Geometry check sheet. Reference: the model listing, model coordinates, mm. A direction names the side the tool comes from. Coordinates: 2 decimals unless noted, no trailing zeros. Write each loop counter-clockwise with the first axis right and the second up, starting at its lowest first coordinate (ties: lowest second). Pieces come first, ordered by that corner, then holes. Notation, with made-up numbers: M 35.25,-25.5 L 88.25,-25.5 A19 cw 88.25,11.5 Z; hole C 67.5,-22.5 d1. An arc over 180 degrees is marked long. Write each question's results on one line, items separated by ' | '.
```python
from build123d import *

# Parameters (mm, degrees)
F0_W     = 85.6
F0_H     = 54
F0_R     = 1.45
F0_R_2   = 0.825
F0_R_3   = 0.445
F0_R_4   = 1.625
F0_R_5   = 1.15
F0_R_6   = 0.875
F0_R_7   = 0.46
F0_R_8   = 0.8
F1_DEPTH = 1.5
F3_DEPTH = 13
F4_R     = 4.15
F4_R_2   = 1.7
F5_DEPTH = 9.5
F6_R     = 0.5


with BuildPart() as f1:
    # F0 (on Top) → F1 (new body)
    with BuildSketch(Plane.XY):
        Rectangle(F0_W, F0_H)
        with Locations((-17.3, -9)):
            Circle(F0_R, mode=Mode.SUBTRACT)
        with Locations((30.375, -24.555)):
            Circle(F0_R_2, mode=Mode.SUBTRACT)
        with Locations((27.075, -21.255)):
            Circle(F0_R_3, mode=Mode.SUBTRACT)
        with Locations((33.425, -22.525)):
            Circle(F0_R_4, mode=Mode.SUBTRACT)
        with Locations((24.535, -19.985)):
            Circle(F0_R_3, mode=Mode.SUBTRACT)
        with Locations((24.535, -17.445)):
            Circle(F0_R_3, mode=Mode.SUBTRACT)
        with Locations((27.075, -18.715)):
            Circle(F0_R_3, mode=Mode.SUBTRACT)
        with Locations((24.535, -14.905)):
            Circle(F0_R_3, mode=Mode.SUBTRACT)
        with Locations((27.075, -16.175)):
            Circle(F0_R_3, mode=Mode.SUBTRACT)
        with Locations((27.075, -13.635)):
            Circle(F0_R_3, mode=Mode.SUBTRACT)
        with Locations((24.535, -12.365)):
            Circle(F0_R_3, mode=Mode.SUBTRACT)
        with Locations((30.375, -9.065)):
            Circle(F0_R_2, mode=Mode.SUBTRACT)
        with Locations((33.425, -11.095)):
            Circle(F0_R_4, mode=Mode.SUBTRACT)
        with Locations((32.65, -3.04)):
            Circle(F0_R_5, mode=Mode.SUBTRACT)
        with Locations((38.33, -3.04)):
            Circle(F0_R_5, mode=Mode.SUBTRACT)
        with Locations((-40.425, 23.375)):
            Circle(F0_R_6, mode=Mode.SUBTRACT)
        with Locations((-38.175, 23.375)):
            Circle(F0_R_6, mode=Mode.SUBTRACT)
        with Locations((-35.925, 23.375)):
            Circle(F0_R_6, mode=Mode.SUBTRACT)
        with Locations((-33.675, 23.375)):
            Circle(F0_R_6, mode=Mode.SUBTRACT)
        with Locations((-40.425, 25.625)):
            Circle(F0_R_6, mode=Mode.SUBTRACT)
        with Locations((-38.175, 25.625)):
            Circle(F0_R_6, mode=Mode.SUBTRACT)
        with Locations((-35.925, 25.625)):
            Circle(F0_R_6, mode=Mode.SUBTRACT)
        with Locations((-33.675, 25.625)):
            Circle(F0_R_6, mode=Mode.SUBTRACT)
        with Locations((-31.425, 23.375)):
            Circle(F0_R_6, mode=Mode.SUBTRACT)
        with Locations((-29.175, 23.375)):
            Circle(F0_R_6, mode=Mode.SUBTRACT)
        with Locations((-26.925, 23.375)):
            Circle(F0_R_6, mode=Mode.SUBTRACT)
        with Locations((-24.675, 23.375)):
            Circle(F0_R_6, mode=Mode.SUBTRACT)
        with Locations((-22.425, 23.375)):
            Circle(F0_R_6, mode=Mode.SUBTRACT)
        with Locations((-31.425, 25.625)):
            Circle(F0_R_6, mode=Mode.SUBTRACT)
        with Locations((-29.175, 25.625)):
            Circle(F0_R_6, mode=Mode.SUBTRACT)
        with Locations((-26.925, 25.625)):
            Circle(F0_R_6, mode=Mode.SUBTRACT)
        with Locations((-24.675, 25.625)):
            Circle(F0_R_6, mode=Mode.SUBTRACT)
        with Locations((-22.425, 25.625)):
            Circle(F0_R_6, mode=Mode.SUBTRACT)
        with Locations((-20.175, 23.375)):
            Circle(F0_R_6, mode=Mode.SUBTRACT)
        with Locations((-17.925, 23.375)):
            Circle(F0_R_6, mode=Mode.SUBTRACT)
        with Locations((-15.675, 23.375)):
            Circle(F0_R_6, mode=Mode.SUBTRACT)
        with Locations((-13.425, 23.375)):
            Circle(F0_R_6, mode=Mode.SUBTRACT)
        with Locations((-20.175, 25.625)):
            Circle(F0_R_6, mode=Mode.SUBTRACT)
        with Locations((-17.925, 25.625)):
            Circle(F0_R_6, mode=Mode.SUBTRACT)
        with Locations((-15.675, 25.625)):
            Circle(F0_R_6, mode=Mode.SUBTRACT)
        with Locations((-13.425, 25.625)):
            Circle(F0_R_6, mode=Mode.SUBTRACT)
        with Locations((33.01, 0.03)):
            Circle(F0_R_7, mode=Mode.SUBTRACT)
        with Locations((35.63, 0.03)):
            Circle(F0_R_7, mode=Mode.SUBTRACT)
        with Locations((33.01, 2.53)):
            Circle(F0_R_7, mode=Mode.SUBTRACT)
        with Locations((35.63, 2.53)):
            Circle(F0_R_7, mode=Mode.SUBTRACT)
        with Locations((33.01, 4.53)):
            Circle(F0_R_7, mode=Mode.SUBTRACT)
        with Locations((35.63, 4.53)):
            Circle(F0_R_7, mode=Mode.SUBTRACT)
        with Locations((33.01, 7.03)):
            Circle(F0_R_7, mode=Mode.SUBTRACT)
        with Locations((35.63, 7.03)):
            Circle(F0_R_7, mode=Mode.SUBTRACT)
        with Locations((32.65, 10.1)):
            Circle(F0_R_5, mode=Mode.SUBTRACT)
        with Locations((38.33, 10.1)):
            Circle(F0_R_5, mode=Mode.SUBTRACT)
        with BuildLine():
            Line((2.425, 18.3), (2.425, 16.3))
            ThreePointArc((2.425, 16.3), (1.05, 14.925), (-0.325, 16.3))
            Line((-0.325, 16.3), (-0.325, 18.3))
            ThreePointArc((-0.325, 18.3), (1.05, 19.675), (2.425, 18.3))
        make_face(mode=Mode.SUBTRACT)
        with BuildLine():
            ThreePointArc((7.175, 18.3), (8.55, 19.675), (9.925, 18.3))
            Line((9.925, 18.3), (9.925, 16.3))
            ThreePointArc((9.925, 16.3), (8.55, 14.925), (7.175, 16.3))
            Line((7.175, 16.3), (7.175, 18.3))
        make_face(mode=Mode.SUBTRACT)
        with Locations((18.2, 19)):
            Circle(F0_R_8, mode=Mode.SUBTRACT)
        with Locations((20.7, 19)):
            Circle(F0_R_8, mode=Mode.SUBTRACT)
        with BuildLine():
            Line((3.8, 22.5), (5.8, 22.5))
            ThreePointArc((5.8, 22.5), (7.3, 21), (5.8, 19.5))
            Line((5.8, 19.5), (3.8, 19.5))
            ThreePointArc((3.8, 19.5), (2.3, 21), (3.8, 22.5))
        make_face(mode=Mode.SUBTRACT)
        with Locations((18.2, 24)):
            Circle(F0_R_8, mode=Mode.SUBTRACT)
        with Locations((23.2, 19)):
            Circle(F0_R_8, mode=Mode.SUBTRACT)
        with Locations((25.7, 19)):
            Circle(F0_R_8, mode=Mode.SUBTRACT)
        with Locations((28.2, 19)):
            Circle(F0_R_8, mode=Mode.SUBTRACT)
        with Locations((37.8, 14.5)):
            Circle(F0_R, mode=Mode.SUBTRACT)
        with Locations((23.2, 24)):
            Circle(F0_R_8, mode=Mode.SUBTRACT)
        with Locations((28.2, 24)):
            Circle(F0_R_8, mode=Mode.SUBTRACT)
    extrude(amount=F1_DEPTH)

    # F2 (on face) → F3 (join)
    with BuildSketch(Plane.XY.offset(1.5)):
        with BuildLine():
            ThreePointArc((2.425, 16.3), (2.1694873279, 15.5016434865), (1.4979118217, 15))
            Line((1.4979118217, 15), (8.1020881783, 15))
            ThreePointArc((8.1020881783, 15), (7.4305126721, 15.5016434865), (7.175, 16.3))
            Line((7.175, 16.3), (7.175, 18.3))
            ThreePointArc((7.175, 18.3), (8.256849015, 19.6433865788), (9.8, 18.8728219619))
            Line((9.8, 18.8728219619), (9.8, 25))
            Line((9.8, 25), (-0.2, 25))
            Line((-0.2, 25), (-0.2, 18.8728219619))
            ThreePointArc((-0.2, 18.8728219619), (1.343150985, 19.6433865788), (2.425, 18.3))
            Line((2.425, 18.3), (2.425, 16.3))
        make_face()
        with BuildLine():
            ThreePointArc((3.8, 19.5), (2.3, 21), (3.8, 22.5))
            Line((3.8, 22.5), (5.8, 22.5))
            ThreePointArc((5.8, 22.5), (7.3, 21), (5.8, 19.5))
            Line((5.8, 19.5), (3.8, 19.5))
        make_face(mode=Mode.SUBTRACT)
        with BuildLine():
            Line((5.8, 22.5), (3.8, 22.5))
            ThreePointArc((3.8, 22.5), (2.3, 21), (3.8, 19.5))
            Line((3.8, 19.5), (5.8, 19.5))
            ThreePointArc((5.8, 19.5), (7.3, 21), (5.8, 22.5))
        make_face()
        with BuildLine():
            ThreePointArc((7.175, 16.3), (7.4305126721, 15.5016434865), (8.1020881783, 15))
            Line((8.1020881783, 15), (8.9979118217, 15))
            ThreePointArc((8.9979118217, 15), (9.4735383659, 15.2813234632), (9.8, 15.7271780381))
            Line((9.8, 15.7271780381), (9.8, 18.8728219619))
            ThreePointArc((9.8, 18.8728219619), (8.256849015, 19.6433865788), (7.175, 18.3))
            Line((7.175, 18.3), (7.175, 16.3))
        make_face()
        with BuildLine():
            ThreePointArc((-0.2, 15.7271780381), (0.1264616341, 15.2813234632), (0.6020881783, 15))
            Line((0.6020881783, 15), (1.4979118217, 15))
            ThreePointArc((1.4979118217, 15), (2.1694873279, 15.5016434865), (2.425, 16.3))
            Line((2.425, 16.3), (2.425, 18.3))
            ThreePointArc((2.425, 18.3), (1.343150985, 19.6433865788), (-0.2, 18.8728219619))
            Line((-0.2, 18.8728219619), (-0.2, 15.7271780381))
        make_face()
        with BuildLine():
            Line((-0.2, 15.7271780381), (-0.2, 15))
            Line((-0.2, 15), (0.6020881783, 15))
            ThreePointArc((0.6020881783, 15), (0.1264616341, 15.2813234632), (-0.2, 15.7271780381))
        make_face()
        with BuildLine():
            ThreePointArc((9.8, 15.7271780381), (9.4735383659, 15.2813234632), (8.9979118217, 15))
            Line((8.9979118217, 15), (9.8, 15))
            Line((9.8, 15), (9.8, 15.7271780381))
        make_face()
    extrude(amount=F3_DEPTH)

    # F4 (on face) → F5 (join)
    with BuildSketch(Plane(origin=(0, 25, 0), x_dir=(-1, 0, 0), z_dir=(0, 1, 0))):
        with Locations((-4.8, 9.5)):
            Circle(F4_R)
        with Locations((-4.8, 9.5)):
            Circle(F4_R_2, mode=Mode.SUBTRACT)
    extrude(amount=F5_DEPTH)

    # F6
    f6_edges = [f1.edges().sort_by_distance(p)[0] for p in [
        (8.95, 34.5, 9.5),
    ]]
    fillet(f6_edges, radius=F6_R)


solid = f1.part
```
Q1. Sectioned sample at B-B on z = 4.25. Record the cut outline in (x, y).
Geometry check:
outline: M -0.2,15 L 9.8,15 L 9.8,25 L -0.2,25 Z
Q2. Scan lines: probe 1 along Y at (x, z) = (18.2, 0.65); probe 2 along X at (y, z) = (27.5, 9.25); probe 3 along Z at (x, y) = (-15.5, -15.5). Record each from-to range of solid material in increasing order.
Geometry check:
probe 1: y = -27 to 18.2, 19.8 to 23.2, 24.8 to 27 | probe 2: x = 0.66 to 3.12, 6.48 to 8.94 | probe 3: z = 0 to 1.5
Q3. Sectioned sample at C-C on y = 28. Record the cut outline in (x, z).
Geometry check:
outline: C 4.8,9.5 d8.3; hole C 4.8,9.5 d3.4
Q4. Access from +Z, -Z, +X, -X, +Y, -Y to the whole of each face (thin tool, end or side, straight path). Record for faces 1 (the flat face through (9.8, 20, 8)), 2 (the cylindrical face through (-15.86, 22.52, 0.74)).
Geometry check:
face 1: +Z, +X, +Y, -Y | face 2: +Z, -Z
Q5. Sectioned sample at A-A on x = -9.5. Record the cut outline in (y, z).
Geometry check:
outline: M -27,0 L 27,0 L 27,1.5 L -27,1.5 Z
Q6. Mould release check, pull along Y, two halves, no side actions. Record for faces 3 (the flat face through (5, 25, 9)), 4 (the cylindrical face through (-36.619, 22.843, 0.74)), 5 (the flat face through (5, 20, 14.5)): pulls with the +Y half, pulls with the -Y half, needs draft (parallel to the pull), parting line crosses it, or undercut.
Geometry check:
face 3: pulls with the +Y half | face 4: undercut | face 5: needs draft
Q7. Depth check by flat-ended pin: P1, Ø1.6, axis at x = -13.425, y = 23.375, coming from the +Z side; P2, Ø3, axis at x = -20.175, y = 23.375, coming from the +Z side; P3, Ø8, axis at x = 10, z = 12, coming from the -Y side; P4, Ø1.6, axis at x = 5, z = 1, coming from the +Y side. Enter the tip coordinate at first touch or a pass-through.
Geometry check:
P1: passes through | P2: stops at z = 1.5 | P3: stops at y = 15 | P4: stops at y = 27
